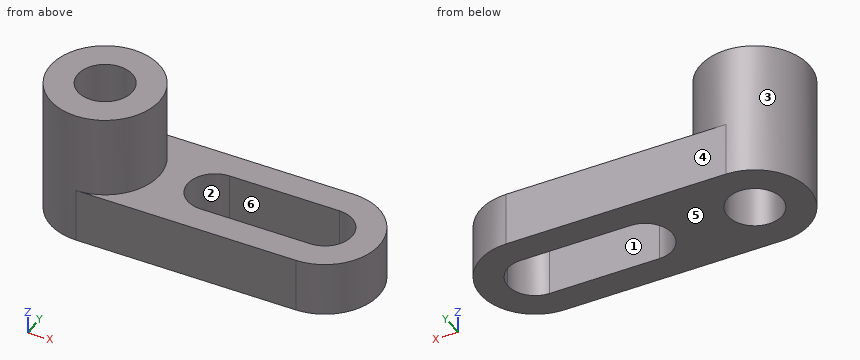
from build123d import *

# Parameters (mm, degrees)
F1_DEPTH  = 25.4
F2_R      = 6.35
F3_DEPTH  = 38.1
F5_DEPTH  = 25.4
F7_DEPTH  = 25.4
F8_DEPTH  = 25.4
F9_DEPTH  = 25.4
F11_DEPTH = 25.4
F12_DEPTH = 19.05


with BuildPart() as f1:
    # F0 (on Front) → F1 (new body)
    with BuildSketch(Plane.XZ):
        Polygon((-37.6096788886, 50.8), (-75.7096788886, 50.8), (-75.7096788886, 0), (13.1903211114, 0), (13.1903211114, 12.7), (-37.6096788886, 12.7), align=None)
    extrude(amount=F1_DEPTH)

    # F2 (on face) → F3 (cut)
    with BuildSketch(Plane.XY.offset(50.8)):
        with BuildLine():
            ThreePointArc((-56.6596788886, 0), (-47.6794227675, -3.7197438789), (-43.9596788886, -12.7))
            ThreePointArc((-43.9596788886, -12.7), (-47.6794227675, -21.6802561211), (-56.6596788886, -25.4))
            Line((-56.6596788886, -25.4), (-37.6096788886, -25.4))
            Line((-37.6096788886, -25.4), (-37.6096788886, 0))
            Line((-37.6096788886, 0), (-56.6596788886, 0))
        make_face()
        with Locations((-56.6596788886, -12.7)):
            Circle(F2_R)
    extrude(amount=-F3_DEPTH, mode=Mode.SUBTRACT)

    # F4 (on face) → F5 (cut)
    with BuildSketch(Plane.XZ.offset(25.4)):
        with BuildLine():
            ThreePointArc((-74.1441026044, 0), (-75.2174849859, 1.8027068987), (-75.7096788886, 3.842228181))
            Line((-75.7096788886, 3.842228181), (-75.7096788886, 0))
            Line((-75.7096788886, 0), (-74.1441026044, 0))
        make_face()
    extrude(amount=-F5_DEPTH, mode=Mode.SUBTRACT)

    # F6 (on face) → F7 (cut)
    with BuildSketch(Plane.XY.offset(50.8)):
        with BuildLine():
            ThreePointArc((-56.6596788886, -25.4), (-69.3596788886, -12.7), (-56.6596788886, 0))
            Line((-56.6596788886, 0), (-75.7096788886, 0))
            Line((-75.7096788886, 0), (-75.7096788886, -25.4))
            Line((-75.7096788886, -25.4), (-56.6596788886, -25.4))
        make_face()
    extrude(amount=-F7_DEPTH, mode=Mode.SUBTRACT)

    # F8 (cut): a face of the model
    f8_faces = [f1.faces().sort_by_distance(p)[0] for p in [
        (-70.7292854187, -12.7, 25.4),
    ]]
    extrude(f8_faces, amount=-F8_DEPTH, mode=Mode.SUBTRACT)

    # F9 (cut): a face of the model
    f9_faces = [f1.faces().sort_by_distance(p)[0] for p in [
        (-56.6596788886, -12.7, 12.7),
    ]]
    extrude(f9_faces, amount=-F9_DEPTH, mode=Mode.SUBTRACT)

    # F10 (on face) → F11 (cut)
    with BuildSketch(Plane.XY.offset(12.7)):
        with BuildLine():
            ThreePointArc((-31.2596788886, -19.05), (-26.7695508281, -17.1901280605), (-24.9096788886, -12.7))
            ThreePointArc((-24.9096788886, -12.7), (-26.7695508281, -8.2098719395), (-31.2596788886, -6.35))
            ThreePointArc((-31.2596788886, -6.35), (-37.6096788886, -12.7), (-31.2596788886, -19.05))
        make_face()
        with BuildLine():
            ThreePointArc((-31.2596788886, -6.35), (-26.7695508281, -8.2098719395), (-24.9096788886, -12.7))
            ThreePointArc((-24.9096788886, -12.7), (-26.7695508281, -17.1901280605), (-31.2596788886, -19.05))
            Line((-31.2596788886, -19.05), (-5.8596788886, -19.05))
            ThreePointArc((-5.8596788886, -19.05), (-12.2096788886, -12.7), (-5.8596788886, -6.35))
            Line((-5.8596788886, -6.35), (-31.2596788886, -6.35))
        make_face()
        with BuildLine():
            ThreePointArc((0.4903211114, -12.7), (-1.3695508281, -8.2098719395), (-5.8596788886, -6.35))
            ThreePointArc((-5.8596788886, -6.35), (-12.2096788886, -12.7), (-5.8596788886, -19.05))
            ThreePointArc((-5.8596788886, -19.05), (-1.3695508281, -17.1901280605), (0.4903211114, -12.7))
        make_face()
        with BuildLine():
            ThreePointArc((-5.8596788886, 0), (6.8403211114, -12.7), (-5.8596788886, -25.4))
            Line((-5.8596788886, -25.4), (13.1903211114, -25.4))
            Line((13.1903211114, -25.4), (13.1903211114, 0))
            Line((13.1903211114, 0), (-5.8596788886, 0))
        make_face()
    extrude(amount=-F11_DEPTH, mode=Mode.SUBTRACT)

    # F12 (cut): a face of the model
    f12_faces = [f1.faces().sort_by_distance(p)[0] for p in [
        (-56.6596788886, -0.3592102448, 50.8),
    ]]
    extrude(f12_faces, amount=-F12_DEPTH, mode=Mode.SUBTRACT)


solid = f1.part
For this review, take the finished solid that the model builds, in its own axes (mm). Face numbers are marked on the shaded views. A direction names the side the tool comes from. Round coordinates to 2 decimals unless told otherwise and drop trailing zeros. Loops run counter-clockwise (first coordinate to the right, second up) from the corner with the lowest first, then second, coordinate; pieces in that order, holes last. Notation, with made-up numbers: (84.25, -29.75) - (127.25, -29.75) arc R23 cw to (127.25, 1.25) - close; hole circle Ø1 at (38.5, 73). An arc over 180 degrees is marked (long way). Use one line per item in the form item = value.
Item 1: Clearance check with flat-ended pins moving along their axes: P1, Ø1, axis at x = -26.5, z = 14.5, coming from the -Y side; P2, Ø1, axis at y = -3, z = 22, coming from the -X side; P3, Ø12.5, axis at x = -12.5, y = -13.5, coming from the +Z side. State where each tip first meets the part, or that it passes through.
Answers:
P1 = through
P2 = -65.41
P3 = 12.7
Item 2: Mouldability with a two-part tool opening along Y and no side actions: class the marked faces 1, 2, 3 and 4 as +Y half, -Y half, draft (parallel to the pull), parting line (faces both ways), or undercut.
Answers:
face_1 = undercut
face_2 = undercut
face_3 = parting line
face_4 = +Y half
Item 3: For line 1 (X direction, y = -11, z = 2); line 2 (Y direction, x = -29.5, z = 2); line 3 (X direction, y = -7.25, z = 7.5), list the stretches that pass through material, from the lowest coordinate up.
Answers:
line_1 = -69.25 to -62.78, -50.54 to -37.38, 0.26 to 6.73
line_2 = -25.4 to -19.05, -6.35 to 0
line_3 = -68.13 to -59.92, -53.4 to -34.52, -2.6 to 5.61
Item 4: Consider section D-D on z = 23. Write out the cut boundary in (x, y).
Answers:
outline = circle Ø25.4 at (-56.66, -12.7); hole circle Ø12.7 at (-56.66, -12.7)
Item 5: Consider section C-C on y = -18. Write out the cut boundary in (x, z), then the cut area to 3 significant figures.
Answers:
outline = (-68.2, 0) - (-60.16, 0) - (-60.16, 31.75) - (-68.2, 31.75) - close; (-53.16, 0) - (-34.76, 0) - (-34.76, 12.7) - (-45.12, 12.7) - (-45.12, 31.75) - (-53.16, 31.75) - close; (-2.36, 0) - (5.68, 0) - (5.68, 12.7) - (-2.36, 12.7) - close
area = 745 mm^2
Item 6: Consider section A-A on x = -24. Write out the cut boundary in (y, z).
Answers:
outline = (-25.4, 0) - (-19.05, 0) - (-19.05, 12.7) - (-25.4, 12.7) - close; (-6.35, 0) - (0, 0) - (0, 12.7) - (-6.35, 12.7) - close
Item 7: Consider section B-B on z = 3.5. Write out the cut boundary in (x, y), then the cut area to 3 significant figures.
Answers:
outline = (-56.66, -25.4) - (-5.86, -25.4) arc R12.7 ccw to (-5.86, 0) - (-56.66, 0) arc R12.7 ccw to start; hole circle Ø12.7 at (-56.66, -12.7); hole (-31.26, -19.05) - (-5.86, -19.05) arc R6.35 ccw to (-5.86, -6.35) - (-31.26, -6.35) arc R6.35 ccw to start
area = 1,220 mm^2
Item 8: Tool access review of the marked faces 5 and 6: name each direction out of +Z, -Z, +X, -X, +Y, -Y from which nothing blocks a thin tool from reaching the whole face with its end or side.
Answers:
face_5 = -Z, +X, -X, +Y, -Y
face_6 = +Z, -Z
